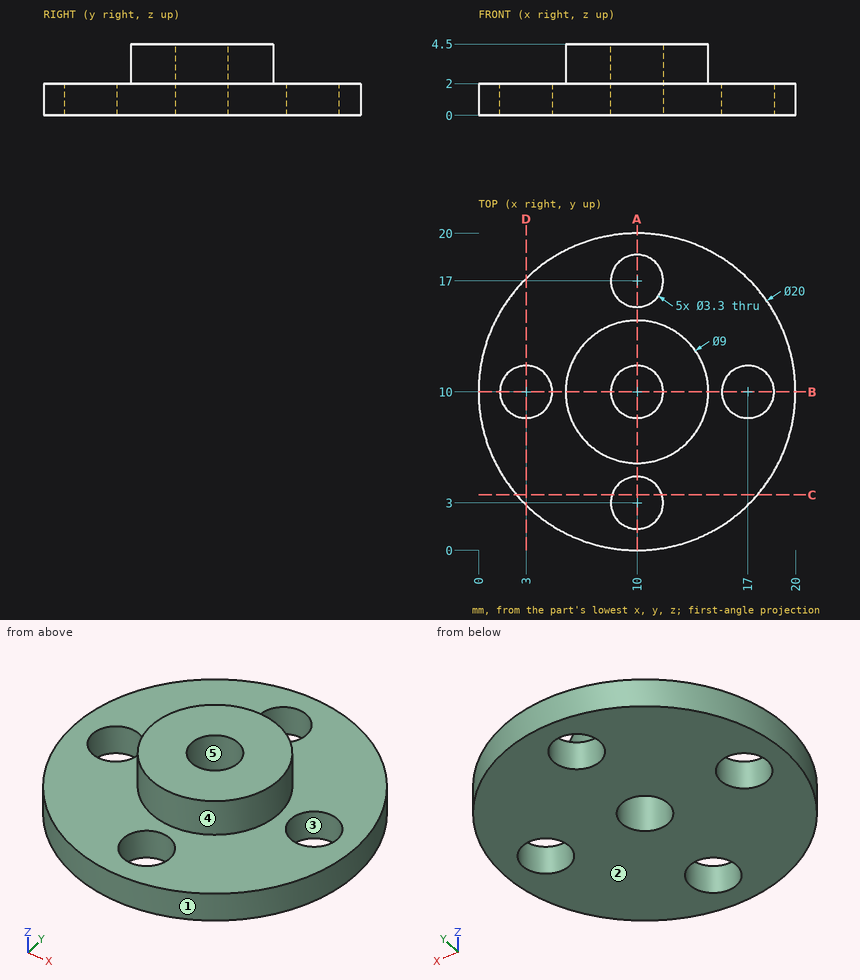
Study the drawing (mm; zero at the part's minimum x, y, z) and answer. A direction names the side the tool comes from. Give positions to 0.01 mm unless a question says otherwise; leave off trailing zeros. Loops run counter-clockwise (first coordinate to the right, second up) from the corner with the lowest first, then second, coordinate; pieces in that order, holes last. Notation, with made-up numbers: M -38.75,-16 L 15.25,-16 A23 cw 15.25,13 Z; hole C 82.25,-22 d2. An arc over 180 degrees is marked long. One line per item, written item: value. Start each with the question number.
1. Find section C-C (y = 3.5). Give the vertices of the cut face in (x, z), and give its area (3 significant figures).
2. This flat-tipped pin is pushed along its axis until it touches: P1, Ø4, axis at x = 3, y = 10, coming from the +Z side. Where does it stop, or does it pass through?
3. Which of the six approach directions +Z, -Z, +X, -X, +Y, -Y give full straight-line access (tool end or side, diameter ignored) to the marked faces 4 and 5?
4. Find section D-D (x = 3). Give the vertices of the cut face in (y, z).
5. Determine the mould class of the marked faces 1, 2 and 3 for opening direction Y: released by +Y, released by -Y, zero draft, split by the parting line, or undercut.
6. Find the intervals of material crossed by probe 1 along Y at (x, z) = (10, 0.6); probe 2 along X at (y, z) = (9.5, 1.8); probe 3 along Y at (x, z) = (9.25, 1.25), in increasing order.
7. Find section A-A (x = 10). Give the vertices of the cut face in (y, z).
Reported:
1. outline: M 2.4,0 L 8.43,0 L 8.43,2 L 2.4,2 Z; M 11.57,0 L 17.6,0 L 17.6,2 L 11.57,2 Z
1. area: 24.1 mm²
2. P1: stops at z = 2
3. face 4: +Z
3. face 5: +Z, -Z
4. outline: M 2.86,0 L 8.35,0 L 8.35,2 L 2.86,2 Z; M 11.65,0 L 17.14,0 L 17.14,2 L 11.65,2 Z
5. face 1: split by the parting line
5. face 2: zero draft
5. face 3: undercut
6. probe 1: y = 0 to 1.35, 4.65 to 8.35, 11.65 to 15.35, 18.65 to 20
6. probe 2: x = 0.01 to 1.43, 4.57 to 8.43, 11.57 to 15.43, 18.57 to 19.99
6. probe 3: y = 0.03 to 1.53, 4.47 to 8.53, 11.47 to 15.53, 18.47 to 19.97
7. outline: M 0,0 L 1.35,0 L 1.35,2 L 0,2 Z; M 4.65,0 L 8.35,0 L 8.35,4.5 L 5.5,4.5 L 5.5,2 L 4.65,2 Z; M 11.65,0 L 15.35,0 L 15.35,2 L 14.5,2 L 14.5,4.5 L 11.65,4.5 Z; M 18.65,0 L 20,0 L 20,2 L 18.65,2 Z
